Geometry check sheet. Reference: the model listing, model coordinates, mm. Round coordinates to 2 decimals unless told otherwise and drop trailing zeros.
```python
from build123d import *

# Parameters (mm, degrees)
SZKIC1_R                    = 3.3
SZKIC1_R_2                  = 3.2
SZKIC1_R_3                  = 1.9
DODANIE_WYCI_GNI_CIE1_DEPTH = 3
SKETCH1_R                   = 2.15
CUT_EXTRUDE1_DEPTH          = 7
CHAMFER1_SIZE               = 3
CUT_EXTRUDE2_DEPTH          = 5.5


with BuildPart() as part:
    # Szkic1 → Dodanie-wyciągnięcie1 (new body)
    with BuildSketch(Plane.XY):
        with BuildLine():
            add(Edge.make_bspline(
                [(0, 87), (18.224844976, 86.998612649), (32.288902875, 73.536902698), (46.435034931, 63.912342556)],
                knots=[0, 0, 0, 0, 1, 1, 1, 1], degree=3))
            add(Edge.make_bspline(
                [(82.741916918, 26.884478511), (77.108810651, 44.216907368), (59.959930782, 53.43272413), (46.435034931, 63.912342556)],
                knots=[0, 0, 0, 0, 1, 1, 1, 1], degree=3))
            add(Edge.make_bspline(
                [(82.741916918, 26.884478511), (88.372384286, 9.551192223), (79.915570217, -7.984418835), (75.133464787, -24.412342556)],
                knots=[0, 0, 0, 0, 1, 1, 1, 1], degree=3))
            add(Edge.make_bspline(
                [(51.137316949, -70.384478511), (65.88071079, -59.671061018), (69.346178061, -40.513663074), (75.133464787, -24.412342556)],
                knots=[0, 0, 0, 0, 1, 1, 1, 1], degree=3))
            add(Edge.make_bspline(
                [(51.137316949, -70.384478511), (36.39229218, -81.095651222), (17.10163575, -78.471544919), (0, -79)],
                knots=[0, 0, 0, 0, 1, 1, 1, 1], degree=3))
            add(Edge.make_bspline(
                [(-51.137316949, -70.384478511), (-36.39229218, -81.095651222), (-17.10163575, -78.471544919), (0, -79)],
                knots=[0, 0, 0, 0, 1, 1, 1, 1], degree=3))
            add(Edge.make_bspline(
                [(-51.137316949, -70.384478511), (-65.88071079, -59.671061018), (-69.346178061, -40.513663074), (-75.133464787, -24.412342556)],
                knots=[0, 0, 0, 0, 1, 1, 1, 1], degree=3))
            add(Edge.make_bspline(
                [(-82.741916918, 26.884478511), (-88.372384286, 9.551192223), (-79.915570217, -7.984418835), (-75.133464787, -24.412342556)],
                knots=[0, 0, 0, 0, 1, 1, 1, 1], degree=3))
            add(Edge.make_bspline(
                [(-82.741916918, 26.884478511), (-77.108810651, 44.216907368), (-59.959930782, 53.43272413), (-46.435034931, 63.912342556)],
                knots=[0, 0, 0, 0, 1, 1, 1, 1], degree=3))
            add(Edge.make_bspline(
                [(0, 87), (-18.224844976, 86.998612649), (-32.288902875, 73.536902698), (-46.435034931, 63.912342556)],
                knots=[0, 0, 0, 0, 1, 1, 1, 1], degree=3))
        make_face()
        Circle(SZKIC1_R, mode=Mode.SUBTRACT)
        with Locations((0, 25)):
            Circle(SZKIC1_R_2, mode=Mode.SUBTRACT)
        with Locations((0, 79)):
            Circle(SZKIC1_R_3, mode=Mode.SUBTRACT)
        with Locations((25, 0)):
            Circle(SZKIC1_R_2, mode=Mode.SUBTRACT)
        with Locations((0, -25)):
            Circle(SZKIC1_R_2, mode=Mode.SUBTRACT)
        with Locations((-25, 0)):
            Circle(SZKIC1_R_2, mode=Mode.SUBTRACT)
        with Locations((75.133464787, 24.412342556)):
            Circle(SZKIC1_R_3, mode=Mode.SUBTRACT)
        with Locations((46.435034931, -63.912342556)):
            Circle(SZKIC1_R_3, mode=Mode.SUBTRACT)
        with Locations((-46.435034931, -63.912342556)):
            Circle(SZKIC1_R_3, mode=Mode.SUBTRACT)
        with Locations((-75.133464787, 24.412342556)):
            Circle(SZKIC1_R_3, mode=Mode.SUBTRACT)
        with BuildLine():
            Line((10.030761285, 35.644910387), (12.836496299, 34.733271819))
            ThreePointArc((12.836496299, 34.733271819), (16.426794018, 34.925977845), (18.959522589, 37.477969089))
            Line((18.959522589, 37.477969089), (26.597641156, 54.869351783))
            ThreePointArc((26.597641156, 54.869351783), (26.579203441, 59.736309453), (22.958213542, 62.988393254))
            Line((22.958213542, 62.988393254), (18.450063705, 64.45317993))
            ThreePointArc((18.450063705, 64.45317993), (13.609094442, 63.950553329), (10.733452075, 60.02393928))
            Line((10.733452075, 60.02393928), (6.690421537, 41.464441676))
            ThreePointArc((6.690421537, 41.464441676), (7.239419176, 37.911136888), (10.030761285, 35.644910387))
        make_face(mode=Mode.SUBTRACT)
        with BuildLine():
            Line((29.052350399, 22.952658594), (30.786390001, 20.565957836))
            ThreePointArc((30.786390001, 20.565957836), (33.804271631, 18.611536236), (37.353314904, 19.18744002))
            Line((37.353314904, 19.18744002), (53.755080895, 28.767790725))
            ThreePointArc((53.755080895, 28.767790725), (56.600890412, 32.716079608), (55.582974944, 37.475435132))
            Line((55.582974944, 37.475435132), (52.796785118, 41.310296435))
            ThreePointArc((52.796785118, 41.310296435), (48.584922212, 43.749113313), (43.950472839, 42.262675991))
            Line((43.950472839, 42.262675991), (29.770593443, 29.624160747))
            ThreePointArc((29.770593443, 29.624160747), (28.126161711, 26.426784072), (29.052350399, 22.952658594))
        make_face(mode=Mode.SUBTRACT)
        with BuildLine():
            Line((36.98082083, 1.50380164), (36.98082083, -1.446322739))
            ThreePointArc((36.98082083, -1.446322739), (38.273558162, -4.801349343), (41.483302234, -6.42150869))
            Line((41.483302234, -6.42150869), (60.383798515, -8.311558318))
            ThreePointArc((60.383798515, -8.311558318), (65.006852754, -6.790050378), (66.98082083, -2.341335177))
            Line((66.98082083, -2.341335177), (66.98082083, 2.398814078))
            ThreePointArc((66.98082083, 2.398814078), (65.006852754, 6.847529279), (60.383798515, 8.369037219))
            Line((60.383798515, 8.369037219), (41.483302234, 6.478987591))
            ThreePointArc((41.483302234, 6.478987591), (38.273558162, 4.858828243), (36.98082083, 1.50380164))
        make_face(mode=Mode.SUBTRACT)
        with BuildLine():
            Line((30.787766351, -20.508926139), (29.053726749, -22.895626897))
            ThreePointArc((29.053726749, -22.895626897), (28.127538061, -26.369752375), (29.771969793, -29.56712905))
            Line((29.771969793, -29.56712905), (43.951849189, -42.205644294))
            ThreePointArc((43.951849189, -42.205644294), (48.586298562, -43.692081616), (52.798161469, -41.253264738))
            Line((52.798161469, -41.253264738), (55.584351294, -37.418403435))
            ThreePointArc((55.584351294, -37.418403435), (56.602266762, -32.659047911), (53.756457245, -28.710759028))
            Line((53.756457245, -28.710759028), (37.354691254, -19.130408323))
            ThreePointArc((37.354691254, -19.130408323), (33.805647981, -18.554504539), (30.787766351, -20.508926139))
        make_face(mode=Mode.SUBTRACT)
        with BuildLine():
            Line((12.83872328, -34.677410915), (10.032988266, -35.589049483))
            ThreePointArc((10.032988266, -35.589049483), (7.241646157, -37.855275984), (6.692648518, -41.408580772))
            Line((6.692648518, -41.408580772), (10.735679056, -59.968078377))
            ThreePointArc((10.735679056, -59.968078377), (13.611321423, -63.894692425), (18.452290686, -64.397319026))
            Line((18.452290686, -64.397319026), (22.960440523, -62.93253235))
            ThreePointArc((22.960440523, -62.93253235), (26.581430423, -59.680448549), (26.599868138, -54.813490879))
            Line((26.599868138, -54.813490879), (18.96174957, -37.422108185))
            ThreePointArc((18.96174957, -37.422108185), (16.429020999, -34.870116941), (12.83872328, -34.677410915))
        make_face(mode=Mode.SUBTRACT)
        with BuildLine():
            Line((-10.010383995, -35.589773073), (-12.81611901, -34.678134505))
            ThreePointArc((-12.81611901, -34.678134505), (-16.406416729, -34.870840531), (-18.939145299, -37.422831775))
            Line((-18.939145299, -37.422831775), (-26.577263867, -54.814214469))
            ThreePointArc((-26.577263867, -54.814214469), (-26.558826152, -59.681172139), (-22.937836252, -62.93325594))
            Line((-22.937836252, -62.93325594), (-18.429686416, -64.398042616))
            ThreePointArc((-18.429686416, -64.398042616), (-13.588717152, -63.895416015), (-10.713074786, -59.968801967))
            Line((-10.713074786, -59.968801967), (-6.670044248, -41.409304362))
            ThreePointArc((-6.670044248, -41.409304362), (-7.219041887, -37.855999574), (-10.010383995, -35.589773073))
        make_face(mode=Mode.SUBTRACT)
        with BuildLine():
            Line((-29.03197311, -22.89752128), (-30.766012712, -20.510820522))
            ThreePointArc((-30.766012712, -20.510820522), (-33.783894342, -18.556398922), (-37.332937615, -19.132302706))
            Line((-37.332937615, -19.132302706), (-53.734703606, -28.712653412))
            ThreePointArc((-53.734703606, -28.712653412), (-56.580513122, -32.660942294), (-55.562597655, -37.420297818))
            Line((-55.562597655, -37.420297818), (-52.776407829, -41.255159121))
            ThreePointArc((-52.776407829, -41.255159121), (-48.564544923, -43.693975999), (-43.930095549, -42.207538678))
            Line((-43.930095549, -42.207538678), (-29.750216154, -29.569023433))
            ThreePointArc((-29.750216154, -29.569023433), (-28.105784422, -26.371646758), (-29.03197311, -22.89752128))
        make_face(mode=Mode.SUBTRACT)
        with BuildLine():
            Line((-36.96044354, -1.448664326), (-36.96044354, 1.501460053))
            ThreePointArc((-36.96044354, 1.501460053), (-38.253180873, 4.856486657), (-41.462924945, 6.476646004))
            Line((-41.462924945, 6.476646004), (-60.363421226, 8.366695632))
            ThreePointArc((-60.363421226, 8.366695632), (-64.986475465, 6.845187692), (-66.96044354, 2.396472491))
            Line((-66.96044354, 2.396472491), (-66.96044354, -2.343676764))
            ThreePointArc((-66.96044354, -2.343676764), (-64.986475465, -6.792391965), (-60.363421226, -8.313899905))
            Line((-60.363421226, -8.313899905), (-41.462924945, -6.423850277))
            ThreePointArc((-41.462924945, -6.423850277), (-38.253180873, -4.80369093), (-36.96044354, -1.448664326))
        make_face(mode=Mode.SUBTRACT)
        with BuildLine():
            Line((-30.767389062, 20.564063452), (-29.03334946, 22.95076421))
            ThreePointArc((-29.03334946, 22.95076421), (-28.107160772, 26.424889688), (-29.751592504, 29.622266363))
            Line((-29.751592504, 29.622266363), (-43.9314719, 42.260781608))
            ThreePointArc((-43.9314719, 42.260781608), (-48.565921273, 43.747218929), (-52.777784179, 41.308402052))
            Line((-52.777784179, 41.308402052), (-55.563974005, 37.473540749))
            ThreePointArc((-55.563974005, 37.473540749), (-56.581889472, 32.714185224), (-53.736079956, 28.765896342))
            Line((-53.736079956, 28.765896342), (-37.334313965, 19.185545636))
            ThreePointArc((-37.334313965, 19.185545636), (-33.785270692, 18.609641852), (-30.767389062, 20.564063452))
        make_face(mode=Mode.SUBTRACT)
        with BuildLine():
            Line((-12.818345991, 34.732548229), (-10.012610977, 35.644186797))
            ThreePointArc((-10.012610977, 35.644186797), (-7.221268868, 37.910413298), (-6.672271229, 41.463718086))
            Line((-6.672271229, 41.463718086), (-10.715301767, 60.02321569))
            ThreePointArc((-10.715301767, 60.02321569), (-13.590944134, 63.949829739), (-18.431913397, 64.452456339))
            Line((-18.431913397, 64.452456339), (-22.940063234, 62.987669664))
            ThreePointArc((-22.940063234, 62.987669664), (-26.561053133, 59.735585862), (-26.579490849, 54.868628193))
            Line((-26.579490849, 54.868628193), (-18.941372281, 37.477245499))
            ThreePointArc((-18.941372281, 37.477245499), (-16.40864371, 34.925254255), (-12.818345991, 34.732548229))
        make_face(mode=Mode.SUBTRACT)
    extrude(amount=DODANIE_WYCI_GNI_CIE1_DEPTH)

    # Sketch1 → Cut-Extrude1 (cut)
    with BuildSketch(Plane(origin=(0, 0, 0), x_dir=(-1, 0, 0), z_dir=(0, 0, -1))):
        with Locations((-17.67766953, 17.67766953)):
            Circle(SKETCH1_R)
        with Locations((17.67766953, 17.67766953)):
            Circle(SKETCH1_R)
        with Locations((17.67766953, -17.67766953)):
            Circle(SKETCH1_R)
        with Locations((-17.67766953, -17.67766953)):
            Circle(SKETCH1_R)
    extrude(amount=-CUT_EXTRUDE1_DEPTH, mode=Mode.SUBTRACT)

    # Chamfer1
    chamfer1_edges = [part.edges().sort_by_distance(p)[0] for p in [
        (-3.2, 25, 3),
        (21.8, 0, 3),
        (-3.2, -25, 3),
        (-28.2, 0, 3),
    ]]
    chamfer(chamfer1_edges, length=CHAMFER1_SIZE - 0.0001)  # a hair under: the kernel refuses the full size

    # Sketch2 → Cut-Extrude2 (cut)
    with BuildSketch(Plane.XY.offset(3)):
        Polygon((-5.15, 2.973353886), (-5.15, -2.973353886), (0, -5.946707773), (5.15, -2.973353886), (5.15, 2.973353886), (0, 5.946707773), align=None)
    extrude(amount=-CUT_EXTRUDE2_DEPTH, mode=Mode.SUBTRACT)


solid = part.part
```
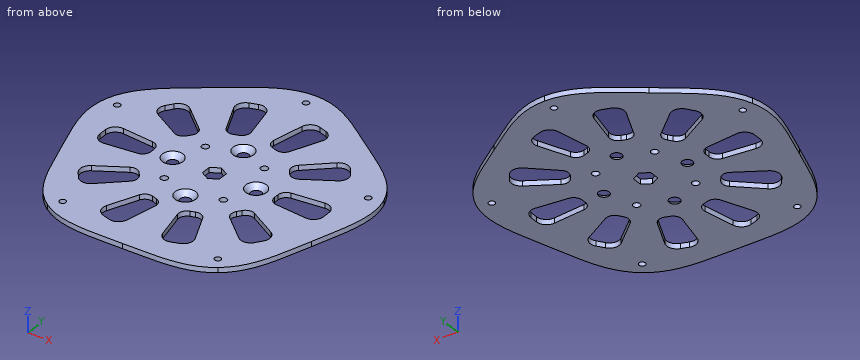
1) Gauge pin test, flat ends, axial feed: pin 1 (6 mm diameter, centred on x = 0, y = 25, fed in from +Z); pin 2 (0.9 mm diameter, centred on y = 0, z = 1, fed in from +X); pin 3 (1 mm diameter, centred on x = 7, z = 1.5, fed in from +Y); pin 4 (1 mm diameter, centred on y = -20, z = 1, fed in from -X). Record the tip position at first contact, or that the pin passes through.
Report:
pin 1: passes through
pin 2: stops at x = 82.74
pin 3: stops at y = 86.43
pin 4: stops at x = -76.65
2) Scan lines: line 1 along Y through (x, z) = (-17, 0.95); line 2 along Y through (x, z) = (20, 1.55); line 3 along Y through (x, z) = (25, 2.45). Record each from-to range of solid material in increasing order.
Report:
line 1: y = -78.92 to -64.68, -35.19 to -19.72, -15.64 to 15.64, 19.72 to 35.24, 64.73 to 83.15
line 2: y = -78.86 to -63.89, -39.79 to 39.85, 63.95 to 81.72
line 3: y = -78.62 to -61.79, -51.17 to -5.65, 5.65 to 51.23, 61.85 to 78.91
3) Sectioned sample at A-A, the plane y = -48. State how many separate pieces and enclosed holes the cut face has, then the cut area to 3 significant figures.
Report:
separate pieces: 3
enclosed holes: 0
area: 310 mm2
